Verification items for the finished model (mm, model axes). Face numbers are marked on the shaded views. A direction names the side the tool comes from. Give positions to 0.01 mm unless a question says otherwise; leave off trailing zeros. Order: outer loops, then holes, each group sorted by start corner. A loop starts at its lowest first (then second) coordinate and runs counter-clockwise, first axis right, second up. Notation, with made-up numbers: (-13, -11) -> (24, -11) arc R9 ccw to (24, 6) -> close; hole circle Ø4 at (1, -5). An arc over 180 degrees is marked (long way). Write each question's results on one line, items separated by ' | '. Start each with the question number.
1. Cross-section at D-D, the plane x = 30. Enter the section's corners in (y, z).
2. Material ranges on L1, parallel to Y at x = 5, z = 13.5; L2, parallel to Z at x = 17.5, y = 31.25; L3, parallel to Y at x = 9.5, z = 10, recorded low to high. Write a range as from..to.
3. Mould release check, pull along Z, two halves, no side actions. Record for the marked faces 1, 2 and 3: +Z half, -Z half, draft (parallel to the pull), parting line (faces both ways), or undercut.
4. Set-up check for the marked faces 4, 5 and 6: record each of +Z, -Z, +X, -X, +Y, -Y from which the full face is reachable in a straight line by a thin tool's end or side.
5. Cross-section at B-B, the plane x = 17.5. Enter the section's corners in (y, z).
6. Depth check by flat-ended pin: pin 1 Ø3 at (y, z) = (48.92, 24.69) entering from -X; pin 2 Ø4 at (y, z) = (48.5, 1) entering from +X; pin 3 Ø4.5 at (x, z) = (17, 19) entering from +Y; pin 4 Ø2 at (y, z) = (48.92, -3.1) entering from -X. Enter the tip coordinate at first touch or a pass-through.
7. Cross-section at A-A, the plane z = 7.62. Enter the section's corners in (x, y).
8. Cross-section at C-C, the plane y = 8. Enter the section's corners in (x, z).
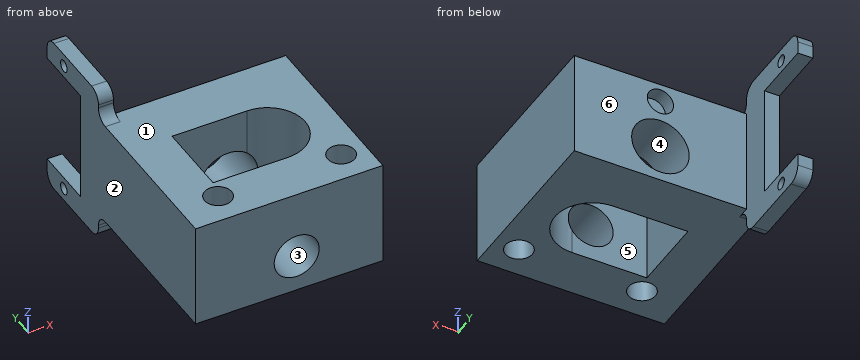
from build123d import *

# Parameters (mm, degrees)
SKETCH2_W            = 35
SKETCH2_H            = 36.068
BOSS_EXTRUDE1_DEPTH  = 21.59
M5_CLEARANCE_HOLE1_D = 5.5
SKETCH13_W           = 22.86
SKETCH13_H           = 15.24
CUT_EXTRUDE3_DEPTH   = 55.699439887
CUT_EXTRUDE1_REACH   = 56.699
SKETCH5_R            = 5.842
BOSS_EXTRUDE2_DEPTH  = 3.048
M2_CLEARANCE_HOLE1_D = 2.4
FILLET2_R            = 2.54
SKETCH11_R           = 2.667
CUT_EXTRUDE2_DEPTH   = 3
SKETCH14_R           = 4.572
CUT_EXTRUDE4_DEPTH   = 64.180572876
FILLET3_R            = 7.62


with BuildPart() as part:
    # Sketch2 → Boss-Extrude1 (new body)
    with BuildSketch(Plane.XY):
        with Locations((17.5, 18.034)):
            Rectangle(SKETCH2_W, SKETCH2_H)
    extrude(amount=BOSS_EXTRUDE1_DEPTH)

    # M5 Clearance Hole1 (through all)
    with Locations(Plane(origin=(0, 0, 0), x_dir=(1, 0, 0), z_dir=(0, 0, -1))):
        with Locations((5, -6.35), (30, -6.35)):
            Hole(M5_CLEARANCE_HOLE1_D / 2)

    # Sketch13 → Cut-Extrude3 (cut, through all)
    with BuildSketch(Plane.XY.offset(21.59)):
        with Locations((17.5, 17.78)):
            Rectangle(SKETCH13_W, SKETCH13_H)
    extrude(amount=-CUT_EXTRUDE3_DEPTH, mode=Mode.SUBTRACT)

    # Sketch5 → Cut-Extrude1 (cut, up to next)
    with BuildSketch(Plane(origin=(0, 36.068, 0), x_dir=(1, 0, 0), z_dir=(0, 1, 0)), mode=Mode.PRIVATE) as cut_extrude1_sk1:
        with Locations(Location((17.5, -7.62, 0), (0, 0, 270))):
            Circle(SKETCH5_R)
    cut_extrude1_tool1 = extrude(cut_extrude1_sk1.sketch, amount=-CUT_EXTRUDE1_REACH, mode=Mode.PRIVATE) & part.part
    add(cut_extrude1_tool1.solids().sort_by_distance((17.5, 36.068, 7.62))[0], mode=Mode.SUBTRACT)

    # Sketch7 → Boss-Extrude2 (add)
    with BuildSketch(Plane.ZY):
        Polygon((-5.715, 55.118), (-5.715, 36.068), (0, 36.068), (0, 0), (21.59, 0), (21.59, 36.068), (27.305, 36.068), (27.305, 55.118), (22.225, 55.118), (22.225, 42.7228), (-0.635, 42.7228), (-0.635, 55.118), align=None)
    extrude(amount=BOSS_EXTRUDE2_DEPTH)

    # M2 Clearance Hole1 (through all)
    with Locations(Plane.ZY.offset(3.048)):
        with Locations((-3.10388, 48.9204), (24.69388, 48.9204)):
            Hole(M2_CLEARANCE_HOLE1_D / 2)

    # Fillet2
    fillet2_edges = [part.edges().sort_by_distance(p)[0] for p in [
        (-1.524, 55.118, -5.715),
        (-1.524, 36.068, -5.715),
        (-1.524, 36.068, 0),
        (-1.524, 36.068, 21.59),
        (-1.524, 36.068, 27.305),
        (-1.524, 55.118, 27.305),
    ]]
    fillet(fillet2_edges, radius=FILLET2_R)

    # Sketch11 → Cut-Extrude2 (cut)
    with BuildSketch(Plane(origin=(0, 36.068, 0), x_dir=(1, 0, 0), z_dir=(0, 1, 0))):
        with Locations(Location((17.5, -17.78, 0), (0, 0, 270))):
            Circle(SKETCH11_R)
    extrude(amount=-CUT_EXTRUDE2_DEPTH, mode=Mode.SUBTRACT)

    # Sketch14 → Cut-Extrude4 (cut, through all)
    with BuildSketch(Plane(origin=(0, 10.16, 0), x_dir=(1, 0, 0), z_dir=(0, 1, 0))):
        with Locations(Location((17.5, -7.62, 0), (0, 0, 270))):
            Circle(SKETCH14_R)
    extrude(amount=-CUT_EXTRUDE4_DEPTH, mode=Mode.SUBTRACT)

    # Fillet3
    # the kernel refuses this fillet: 7.62 mm, written as the material it adds along each edge
    with BuildSketch(Plane(origin=(28.93, 25.4, 21.59), x_dir=(-1, 0, 0), z_dir=(0, 0, -1))) as fillet3_piece_1_section:
        with BuildLine():
            CenterArc((FILLET3_R, -FILLET3_R), FILLET3_R, 90, 90)
            Line((0, -FILLET3_R), (0, 0))
            Line((0, 0), (FILLET3_R, 0))
        make_face()
    fillet3_piece_1 = extrude(amount=21.59, mode=Mode.PRIVATE)
    fillet3_piece_1 = fillet3_piece_1 - Plane(origin=(17.5, 23.659865562, 7.62), x_dir=(0, 0, 1), z_dir=(0, 1, 0)) * Cylinder(5.842, 74, mode=Mode.PRIVATE)
    add(fillet3_piece_1)
    with BuildSketch(Plane(origin=(28.93, 10.16, 21.59), x_dir=(0, 1, 0), z_dir=(0, 0, -1))) as fillet3_piece_2_section:
        with BuildLine():
            CenterArc((FILLET3_R, -FILLET3_R), FILLET3_R, 90, 90)
            Line((0, -FILLET3_R), (0, 0))
            Line((0, 0), (FILLET3_R, 0))
        make_face()
    fillet3_piece_2 = extrude(amount=21.59, mode=Mode.PRIVATE)
    fillet3_piece_2 = fillet3_piece_2 - Plane(origin=(17.5, 11.887502218, 7.62), x_dir=(0, 0, 1), z_dir=(0, 1, 0)) * Cylinder(4.572, 74, mode=Mode.PRIVATE)
    add(fillet3_piece_2)


solid = part.part
Results below:
1) outline: (0, 0) -> (3.6, 0) -> (3.6, 21.59) -> (0, 21.59) -> close; (9.1, 0) -> (36.07, 0) -> (36.07, 21.59) -> (9.1, 21.59) -> close
2) L1: y = 0..3.6, 9.1..36.07 | L2: z = 0..1.78, 13.46..21.59 | L3: y = 0..10.16, 25.4..36.07
3) face 1: +Z half | face 2: draft | face 3: undercut
4) face 4: +Y | face 5: +Z, -Z | face 6: +Z, -Z, +X, +Y
5) outline: (0, 0) -> (10.16, 0) -> (10.16, 3.05) -> (0, 3.05) -> close; (0, 12.19) -> (10.16, 12.19) -> (10.16, 21.59) -> (0, 21.59) -> close; (25.4, 0) -> (36.07, 0) -> (36.07, 1.78) -> (25.4, 1.78) -> close; (25.4, 13.46) -> (36.07, 13.46) -> (36.07, 15.11) -> (33.07, 15.11) -> (33.07, 20.45) -> (36.07, 20.45) -> (36.07, 21.59) -> (25.4, 21.59) -> close
6) pin 1: stops at x = -3.05 | pin 2: stops at x = 0 | pin 3: stops at y = 36.07 | pin 4: passes through
7) outline: (-3.05, 0) -> (12.93, 0) -> (12.93, 10.16) -> (6.07, 10.16) -> (6.07, 25.4) -> (11.66, 25.4) -> (11.66, 36.07) -> (0, 36.07) -> (0, 42.72) -> (-3.05, 42.72) -> close; (22.07, 0) -> (35, 0) -> (35, 36.07) -> (23.34, 36.07) -> (23.34, 25.12) arc R7.62 cw to (22.07, 10.2) -> close; hole circle Ø5.5 at (5, 6.35); hole circle Ø5.5 at (30, 6.35)
8) outline: (-3.05, 0) -> (2.8, 0) -> (2.8, 21.59) -> (-3.05, 21.59) -> close; (7.2, 0) -> (27.8, 0) -> (27.8, 21.59) -> (7.2, 21.59) -> close; (32.2, 0) -> (35, 0) -> (35, 21.59) -> (32.2, 21.59) -> close; hole circle Ø9.14 at (17.5, 7.62)
